```python
from build123d import *

# Parameters (mm, degrees)
BOSS_EXTRUDE12_DEPTH            = 80
CUT_EXTRUDE10_DEPTH             = 114.712356409
CUT_EXTRUDE10_DEPTH_BACK        = 114.712356409
SKETCH37_W                      = 102
SKETCH37_H                      = 56
BOSS_EXTRUDE16_DEPTH            = 3
CUT_EXTRUDE11_DEPTH             = 102.766059637
SKETCH40_W                      = 127.486838651
SKETCH40_H                      = 11.94281061
CUT_EXTRUDE12_DEPTH             = 102.007241851
CUT_EXTRUDE12_DIRECTION_2_REACH = 103.007


with BuildPart() as part:
    # Sketch22 → Boss-Extrude12 (new body)
    with BuildSketch(Plane.XY):
        with BuildLine():
            Line((32.5, -14.5), (-32.5, -14.5))
            ThreePointArc((-32.5, -14.5), (-47, 0), (-32.5, 14.5))
            Line((-32.5, 14.5), (32.5, 14.5))
            ThreePointArc((32.5, 14.5), (47, 0), (32.5, -14.5))
        make_face()
    extrude(amount=BOSS_EXTRUDE12_DEPTH)

    # Sketch35 → Cut-Extrude10 (cut, two sides: drawn at the far end of the back side and taken through both)
    with BuildSketch(Plane(origin=(-32.5, 0, 0), x_dir=(0, 0, -1), z_dir=(1, 0, 0)).offset(-CUT_EXTRUDE10_DEPTH_BACK)):
        Polygon((0, 14.5), (-29.026860374, -14.5), (0, -14.5), align=None)
    extrude(amount=CUT_EXTRUDE10_DEPTH + CUT_EXTRUDE10_DEPTH_BACK, mode=Mode.SUBTRACT)

    # Sketch37 → Boss-Extrude16 (add)
    with BuildSketch(Plane(origin=(0, 7.256711984, 7.249996893), x_dir=(-1, 0, 0), z_dir=(0, -0.7074340219640284, -0.7067793888957138))):
        with Locations((0, -10.26729429)):
            Rectangle(SKETCH37_W, SKETCH37_H)
    extrude(amount=-BOSS_EXTRUDE16_DEPTH)

    # Sketch38 → Cut-Extrude11 (cut, through all)
    with BuildSketch(Plane.XY.offset(80)):
        with BuildLine():
            Line((-32.5, 12.75), (32.5, 12.75))
            ThreePointArc((32.5, 12.75), (45.25, 0), (32.5, -12.75))
            Line((32.5, -12.75), (-32.5, -12.75))
            ThreePointArc((-32.5, -12.75), (-45.25, 0), (-32.5, 12.75))
        make_face()
    extrude(amount=-CUT_EXTRUDE11_DEPTH, mode=Mode.SUBTRACT)

    # Sketch40 → Cut-Extrude12 (cut)
    with BuildSketch(Plane(origin=(0, -12.75, 0), x_dir=(1, 0, 0), z_dir=(0, 1, 0))):
        with Locations((5.984726224, -83.886766037)):
            Rectangle(SKETCH40_W, SKETCH40_H)
    extrude(amount=CUT_EXTRUDE12_DEPTH, mode=Mode.SUBTRACT)

    # Cut-Extrude12 direction 2: up to this face of the body (flat: up to its plane)
    cut_extrude12_direction_2_end = Plane(part.part.faces().sort_by_distance((0, -14.5, 56.635733163))[0])
    # Sketch40 → Cut-Extrude12 direction 2 (cut, up to the picked face)
    with BuildSketch(Plane(origin=(0, -12.75, 0), x_dir=(1, 0, 0), z_dir=(0, 1, 0)), mode=Mode.PRIVATE) as cut_extrude12_direction_2_sk1:
        with Locations((5.984726224, -83.886766037)):
            Rectangle(SKETCH40_W, SKETCH40_H)
    cut_extrude12_direction_2_tool1 = split(extrude(cut_extrude12_direction_2_sk1.sketch, amount=-CUT_EXTRUDE12_DIRECTION_2_REACH, mode=Mode.PRIVATE), bisect_by=cut_extrude12_direction_2_end, keep=Keep.BOTH, mode=Mode.PRIVATE)
    add(cut_extrude12_direction_2_tool1.solids().sort_by(Axis((5.984726, -12.75, 83.886766), (0, -1, 0)))[0], mode=Mode.SUBTRACT)


solid = part.part
```
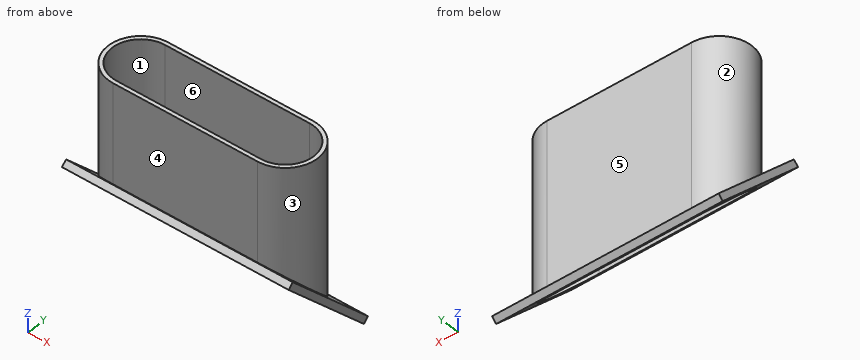
Verification items for the finished model (mm, model axes). Face numbers are marked on the shaded views. A direction names the side the tool comes from. Round coordinates to 2 decimals unless told otherwise and drop trailing zeros. Order: outer loops, then holes, each group sorted by start corner. A loop starts at its lowest first (then second) coordinate and runs counter-clockwise, first axis right, second up. Notation, with made-up numbers: (-18.5, 32.25) - (-3.5, 32.25) arc R9 ccw to (-3.5, 41.25) - close; hole circle Ø10 at (25, 5). An arc over 180 degrees is marked (long way). Use CSV: the item, a comma, the result in double quotes.
(1) Access from +Z, -Z, +X, -X, +Y, -Y to the whole of each face (thin tool, end or side, straight path). Record for the marked faces 5 and 6.
Entries:
face 5,"+Z, +X, -X, +Y"
face 6,"+Z, -Z"
(2) Gauge pin test, flat ends, axial feed: pin 1 Ø10 at (y, z) = (4, 38) entering from -X; pin 2 Ø4 at (y, z) = (4.5, 62.5) entering from -X; pin 3 Ø12 at (x, y) = (4, -2.5) entering from -Z; pin 4 Ø1 at (y, z) = (-5, 38.5) entering from +X. Record the tip position at first contact, or that the pin passes through.
Entries:
pin 1,"x = -47"
pin 2,"x = -46.78"
pin 3,"through"
pin 4,"x = 46.28"
(3) Thickness scan on probe 1 along Y at (x, z) = (0.5, 62); probe 2 along Y at (x, z) = (31.5, 26); probe 3 along X at (y, z) = (1, 36.5). Record the ranges inside material, lowest first. Write a range as from..to.
Entries:
probe 1,"-14.5..-12.75, 12.75..14.5"
probe 2,"12.75..14.5"
probe 3,"-46.97..-45.21, 45.21..46.97"
(4) Section check B-B on z = 50.5. Record the boundary of the cut face in (x, y), and give its area (3 significant figures).
Entries:
outline,"(-32.5, -14.5) - (32.5, -14.5) arc R14.5 ccw to (32.5, 14.5) - (-32.5, 14.5) arc R14.5 ccw to start; hole (-32.5, -12.75) - (32.5, -12.75) arc R12.75 ccw to (32.5, 12.75) - (-32.5, 12.75) arc R12.75 ccw to start"
area,"377 mm^2"
(5) Section check A-A on x = -12. Record the boundary of the cut face in (y, z).
Entries:
outline,"(-19.79, 34.32) - (-12.75, 27.28) - (-12.75, 77.92) - (-14.5, 77.92) - (-14.5, 33.27) - (-17.67, 36.44) - close; (12.75, 1.75) - (19.79, -5.29) - (21.91, -3.17) - (14.5, 4.24) - (14.5, 77.92) - (12.75, 77.92) - close"
(6) Section check C-C on y = -7.5. Record the boundary of the cut face in (x, z).
Entries:
outline,"(-51, 22.02) - (-42.81, 22.02) - (-42.81, 77.92) - (-44.91, 77.92) - (-44.91, 26.26) - (-51, 26.26) - close; (42.81, 22.02) - (51, 22.02) - (51, 26.26) - (44.91, 26.26) - (44.91, 77.92) - (42.81, 77.92) - close"
(7) Mould release check, pull along X, two halves, no side actions. Record for the marked faces 1, 2, 3 and 4: released by +X, released by -X, zero draft, split by the parting line, or undercut.
Entries:
face 1,"undercut"
face 2,"released by -X"
face 3,"released by +X"
face 4,"zero draft"
